Input: part model. Units: mm. Frame: model coordinates. A direction names the side the tool comes from. Coordinates: 2 decimals unless noted, no trailing zeros. Write each loop counter-clockwise with the first axis right and the second up, starting at its lowest first coordinate (ties: lowest second). Pieces come first, ordered by that corner, then holes. Notation, with made-up numbers: M 70,-38.5 L 127,-38.5 A28 cw 127,-7.5 Z; hole C 77.5,-26.75 d6. An arc over 180 degrees is marked long. Use one line per item in the form item = value.
from build123d import *

# Parameters (mm, degrees)
F0_R     = 2.5
F1_DEPTH = 95.25
F2_W     = 6.35
F2_H     = 3.175
F3_DEPTH = 38.101
F4_D     = 4.2
F4_DEPTH = 20
F4_TIP   = 1.2618073


with BuildPart() as f1:
    # F0 (on Top) → F1 (new body)
    with BuildSketch(Plane.XY):
        Polygon((0, 0), (19.05, 0), (38.1, 0), (38.1, 25.4), (19.05, 25.4), (0, 25.4), align=None)
        with Locations((9.525, 12.7)):
            Circle(F0_R, mode=Mode.SUBTRACT)
        with Locations((28.575, 12.7)):
            Circle(F0_R, mode=Mode.SUBTRACT)
        with Locations((9.525, 12.7)):
            Circle(F0_R)
        with Locations((28.575, 12.7)):
            Circle(F0_R)
    extrude(amount=F1_DEPTH)

    # F2 (on face) → F3 (cut, through all)
    with BuildSketch(Plane.YZ.offset(38.1)):
        with Locations((14.2875, 93.6625)):
            Rectangle(F2_W, F2_H)
    extrude(amount=-F3_DEPTH, mode=Mode.SUBTRACT)

    # F4
    with Locations(Plane(origin=(0, 0, 0), x_dir=(1, 0, 0), z_dir=(0, 0, -1))):
        with Locations((9.525, -12.7), (28.575, -12.7)):
            Hole(F4_D / 2, depth=F4_DEPTH)
            with Locations((0, 0, -(F4_DEPTH + F4_TIP / 2))):  # 118° drill point
                Cone(0, F4_D / 2, F4_TIP, mode=Mode.SUBTRACT)


solid = f1.part
(1) First-contact query: pin 1 Ø3 at (x, y) = (10, 15) entering from +Z (3 decimals); pin 2 Ø3.5 at (x, y) = (28.575, 12.7) entering from -Z. Flat tips, straight axial feed; report the tip coordinate or a pass-through.
Computed:
pin_1 = 92.075
pin_2 = 20.21
(2) Section query A-A on z = 14. Return the cut outline in (x, y) (3 decimals).
Computed:
outline = M 0,0 L 38.1,0 L 38.1,25.4 L 0,25.4 Z; hole C 9.525,12.7 d4.2; hole C 28.575,12.7 d4.2
(3) Section query B-B on y = 16. Return the cut outline in (x, z) (3 decimals).
Computed:
outline = M 0,0 L 38.1,0 L 38.1,92.075 L 0,92.075 Z
(4) Set-up query: faces 4 (the cylindrical face through (30.24, 13.98, 10.14)), 5 (the flat face through (19, 11.112, 94)), 6 (the flat face through (38.1, 13, 47)). Return all of +Z, -Z, +X, -X, +Y, -Y with unobstructed straight access to the full face (end or side cutting, diameter ignored); none if empty.
Computed:
face_4 = -Z
face_5 = +Z, +X, -X
face_6 = +Z, -Z, +X, +Y, -Y
(5) Line query: probe 1 along X at (y, z) = (12.7, 11.25) (3 decimals); probe 2 along Z at (x, y) = (25, 16) (3 decimals). Output: solid intervals per line, ascending.
Computed:
probe_1 = 0 to 7.425, 11.625 to 26.475, 30.675 to 38.1
probe_2 = 0 to 92.075
(6) Pull-direction query (Y, two-part tool) for faces 1 (the flat face through (19, 0, 47)), 2 (the flat face through (19, 17.462, 94)), 3 (the flat face through (19, 21, 95.25)); classes: pulls with the +Y half, pulls with the -Y half, needs draft (parallel to the pull), parting line crosses it, or undercut.
Computed:
face_1 = pulls with the -Y half
face_2 = undercut
face_3 = needs draft
